Autodesk Inventor part; units mm, degrees
ref_plane "YZ Plane" through (0, 0, 0) normal (1, 0, 0) x (0, 1, 0)
ref_plane "XZ Plane" through (0, 0, 0) normal (0, 1, 0) x (-1, 0, 0)
ref_plane "XY Plane" through (0, 0, 0) normal (0, 0, 1) x (1, 0, 0)
sketch "Sketch1" plane through (0, 0, 0) normal (0, 0, 1) x (1, 0, 0)
  line L0 (0, 0) -> (165.1, 0)
  line L1 (165.1, 0) -> (165.1, 76.2)
  line L2 (165.1, 76.2) -> (0, 76.2)
  line L3 (0, 76.2) -> (0, 0)
  dimension "d0" = 165.1
  dimension "d1" = 76.2
extrude "Extrusion1" add sketch "Sketch1" along normal blind 6.35
sketch "Sketch3" plane through (0, 0, 6.35) normal (0, 0, 1) x (1, 0, 0)
  line L0 (31.75, 25.4) -> (133.35, 25.4)
  line L1 (0, 0) -> (165.1, 0)
  line L2 (0, 76.2) -> (0, 0)
  dimension "d14" = 101.6
  dimension "d15" = 25.4
  dimension "d16" = 31.75
hole "Hole1" at (31.75, 25.4, 6.35) at (133.35, 25.4, 6.35) direction (0, 0, -1) diameter 4.1656 depth 6.35 tip angle 118 counterbore diameter 7.9502 counterbore depth 2.54
sketch "Sketch4" plane through (0, 0, 0) normal (0, 0, -1) x (-1, 0, 0)
  line L0 (-139.7, 12.7) -> (-25.4, 12.7) construction
  line L1 (-139.7, 9.525) -> (-25.4, 9.525)
  line L2 (-25.4, 15.875) -> (-139.7, 15.875)
  arc A0 (-139.7, 15.875) -> (-139.7, 9.525) centre (-139.7, 12.7) ccw
  arc A1 (-25.4, 9.525) -> (-25.4, 15.875) centre (-25.4, 12.7) ccw
  line L3 (0, 76.2) -> (0, 0)
  line L4 (-139.7, 63.5) -> (-25.4, 63.5) construction
  line L5 (-139.7, 60.325) -> (-25.4, 60.325)
  line L6 (-25.4, 66.675) -> (-139.7, 66.675)
  arc A2 (-139.7, 66.675) -> (-139.7, 60.325) centre (-139.7, 63.5) ccw
  arc A3 (-25.4, 60.325) -> (-25.4, 66.675) centre (-25.4, 63.5) ccw
  line L7 (-165.1, 76.2) -> (0, 76.2)
  point P0 (-82.55, 12.7)
  point P1 (-82.55, 63.5)
  dimension "d24" = 6.35
  dimension "d25" = 25.4
  dimension "d26" = 114.3
  dimension "d27" = 6.35
  dimension "d28" = 50.8
  dimension "d29" = 12.7
  dimension "d32" = 114.3
extrude "Extrusion3" cut sketch "Sketch4" against normal blind 6.35
hole "Hole2" at (31.75, 25.4, 0) direction (0, 0, 1) diameter 9.525 depth 1.5875
hole "Hole4" at (133.35, 25.4, 0) direction (0, 0, 1) diameter 9.525 depth 1.5875
properties part number "bottom"
Check sheet for the modelled part. Datum: model origin and axes. Units: mm. A direction names the side the tool comes from. Round coordinates to 2 decimals unless told otherwise and drop trailing zeros. Loops run counter-clockwise (first coordinate to the right, second up) from the corner with the lowest first, then second, coordinate; pieces in that order, holes last. Notation, with made-up numbers: (51.25, 38.5) - (101.25, 38.5) arc R27 cw to (101.25, 76.5) - close; hole circle Ø9 at (11.5, 75). An arc over 180 degrees is marked (long way). Write item = value, one per line. Start each with the question number.
Q1. Section check D-D (x = 101). Record the boundary of the cut face in (y, z) (3 decimals).
Q2. Thickness scan on L1, parallel to Y at x = 31.75, z = 2.05 (3 decimals); L2, parallel to X at y = 25.4, z = 4.55; L3, parallel to Y at x = 133.35, z = 0.7 (1 decimal). Record the ranges inside material, lowest first.
Q3. Section check B-B (z = 5.25). Record the boundary of the cut face in (x, y) (3 decimals).
Q4. Section check A-A (y = 63.5). Record the boundary of the cut face in (x, z) (3 decimals).
Q5. Release check for a two-part mould opening along Y. For faces 6 (the face through (81, 39, 6.35)), 7 (the face through (82, 66.675, 3)), 8 (the face through (142.874, 63.57, 3.131)), 9 (the face through (81, 0, 3)) record: pulls with the +Y half, pulls with the -Y half, needs draft (parallel to the pull), parting line crosses it, or undercut.
Q6. Section check C-C (y = 25.4). Record the boundary of the cut face in (x, z).
Q7. Depth check by flat-ended pin: P1, Ø7, axis at x = 31.75, y = 25.4, coming from the -Z side. Enter the tip coordinate at first touch or a pass-through.
Q8. Access from +Z, -Z, +X, -X, +Y, -Y to the whole of each face (thin tool, end or side, straight path). Record for faces 1 (the face through (138, 24.37, 0.8)), 2 (the face through (165.1, 38, 3)), 3 (the face through (83, 60.325, 3)), 4 (the face through (0, 39, 3)), 5 (the face through (29.063, 28.33, 5.062)).
Derived:
q1.outline = (0, 0) - (9.525, 0) - (9.525, 6.35) - (0, 6.35) - close; (15.875, 0) - (60.325, 0) - (60.325, 6.35) - (15.875, 6.35) - close; (66.675, 0) - (76.2, 0) - (76.2, 6.35) - (66.675, 6.35) - close
q2.L1 = 0 to 9.525, 15.875 to 23.317, 27.483 to 60.325, 66.675 to 76.2
q2.L2 = 0 to 27.77, 35.73 to 129.37, 137.33 to 165.1
q2.L3 = 0 to 9.5, 15.9 to 20.6, 30.2 to 60.3, 66.7 to 76.2
q3.outline = (0, 0) - (165.1, 0) - (165.1, 76.2) - (0, 76.2) - close; hole (25.4, 9.525) - (139.7, 9.525) arc R3.175 ccw to (139.7, 15.875) - (25.4, 15.875) arc R3.175 ccw to start; hole (25.4, 60.325) - (139.7, 60.325) arc R3.175 ccw to (139.7, 66.675) - (25.4, 66.675) arc R3.175 ccw to start; hole circle Ø7.95 at (31.75, 25.4); hole circle Ø7.95 at (133.35, 25.4)
q4.outline = (0, 0) - (22.225, 0) - (22.225, 6.35) - (0, 6.35) - close; (142.875, 0) - (165.1, 0) - (165.1, 6.35) - (142.875, 6.35) - close
q5.face_6 = needs draft
q5.face_7 = undercut
q5.face_8 = undercut
q5.face_9 = pulls with the -Y half
q6.outline = (0, 0) - (26.99, 0) - (26.99, 1.59) - (29.67, 1.59) - (29.67, 3.81) - (27.77, 3.81) - (27.77, 6.35) - (0, 6.35) - close; (33.83, 1.59) - (36.51, 1.59) - (36.51, 0) - (128.59, 0) - (128.59, 1.59) - (131.27, 1.59) - (131.27, 3.81) - (129.37, 3.81) - (129.37, 6.35) - (35.73, 6.35) - (35.73, 3.81) - (33.83, 3.81) - close; (135.43, 1.59) - (138.11, 1.59) - (138.11, 0) - (165.1, 0) - (165.1, 6.35) - (137.33, 6.35) - (137.33, 3.81) - (135.43, 3.81) - close
q7.P1 = 1.59
q8.face_1 = -Z
q8.face_2 = +Z, -Z, +X, +Y, -Y
q8.face_3 = +Z, -Z
q8.face_4 = +Z, -Z, -X, +Y, -Y
q8.face_5 = +Z
